Check sheet for the modelled part. Datum: model origin and axes. Units: mm. A direction names the side the tool comes from. Give positions to 0.01 mm unless a question says otherwise; leave off trailing zeros. Loops run counter-clockwise (first coordinate to the right, second up) from the corner with the lowest first, then second, coordinate; pieces in that order, holes last. Notation, with made-up numbers: (-40, -38) - (-7, -38) arc R17 cw to (-7, -11) - close; hole circle Ø3 at (80, -12). An arc over 180 degrees is marked (long way). Use one line per item in the form item = value.
from build123d import *

# Parameters (mm, degrees)
F0_W         = 1.8
F0_H         = 50
F0_W_2       = 18.2
F0_W_3       = 1.6
F1_DEPTH     = 1
F2_DEPTH     = 20
F3_DEPTH     = 20
F4_T4_DEPTH  = 76.7042031505
F4_T9_DEPTH  = 76.6048284538
F4_T14_DEPTH = 76.8048284538
F4_T19_DEPTH = 76.7042031505
F4_T24_DEPTH = 76.6048284538
F4_T29_DEPTH = 76.8048284538
F5_R         = 5
F6_R         = 2
F7_R         = 5
F8_SIZE      = 0.5


# Not quite as in the source:
# - a fillet or chamfer that OpenCascade refuses, or shapes differently, is made with other operations: its cross-section is extruded or revolved along the edge and cut away or added


with BuildPart() as f1:
    # F0 (on Top) → F1 (new body)
    with BuildSketch(Plane.XY):
        with Locations((0.9, 25)):
            Rectangle(F0_W, F0_H)
        with Locations((10.9, 25)):
            Rectangle(F0_W_2, F0_H)
        with Locations((20.8, 25)):
            Rectangle(F0_W_3, F0_H)
        with BuildLine():
            Line((21.6, 50), (21.6, 0))
            Line((21.6, 0), (32.3006253033, 0))
            ThreePointArc((32.3006253033, 0), (36.6893218813, 25), (32.3006253033, 50))
            Line((32.3006253033, 50), (21.6, 50))
        make_face()
        with BuildLine():
            ThreePointArc((32.3006253033, 50), (36.6893218813, 25), (32.3006253033, 0))
            Line((32.3006253033, 0), (34, 0))
            ThreePointArc((34, 0), (38.2893218813, 25), (34, 50))
            Line((34, 50), (32.3006253033, 50))
        make_face()
    extrude(amount=F1_DEPTH)

    # F0 (on Top) → F2 (join)
    with BuildSketch(Plane.XY):
        with Locations((0.9, 25)):
            Rectangle(F0_W, F0_H)
        with Locations((20.8, 25)):
            Rectangle(F0_W_3, F0_H)
    extrude(amount=F2_DEPTH)

    # F0 (on Top) → F3 (join)
    with BuildSketch(Plane.XY):
        with BuildLine():
            ThreePointArc((32.3006253033, 50), (36.6893218813, 25), (32.3006253033, 0))
            Line((32.3006253033, 0), (34, 0))
            ThreePointArc((34, 0), (38.2893218813, 25), (34, 50))
            Line((34, 50), (32.3006253033, 50))
        make_face()
    extrude(amount=F3_DEPTH)

    # F4: fillet of radius 15 on 6 edges, made by hand


with BuildPart() as f4_tool2:
    # F4_s3 → F4_t4 (new body)
    with BuildSketch(Plane.YZ.offset(-5.2017889236)):
        with BuildLine():
            ThreePointArc((15.0009656854, 20.0004), (4.3933982822, 15.6066017178), (-0.0004, 4.9990343146))
            Line((-0.0004, 4.9990343146), (-1.5005365685, 4.9990343146))
            ThreePointArc((-1.5005365685, 4.9990343146), (-1.5001365685, 12.4995171573), (-1.5001365685, 20))
            Line((-1.5001365685, 20), (0, 21.5001365685))
            ThreePointArc((0, 21.5001365685), (7.5004828427, 21.5001365685), (15.0009656854, 21.5005365685))
            Line((15.0009656854, 21.5005365685), (15.0009656854, 20.0004))
        make_face()
    extrude(amount=F4_T4_DEPTH)

    split(bisect_by=Plane.YZ.offset(21.6), keep=Keep.TOP)


with BuildPart() as f1_1:
    add(f1.part)

    # F4_t1: cut F4_tool2
    add(f4_tool2.part, mode=Mode.SUBTRACT)


with BuildPart() as f4_tool7:
    # F4_s8 → F4_t9 (new body)
    with BuildSketch(Plane.YZ.offset(-17.5024142269)):
        with BuildLine():
            ThreePointArc((15.0009656854, 20.0004), (4.3933982822, 15.6066017178), (-0.0004, 4.9990343146))
            Line((-0.0004, 4.9990343146), (-1.5005365685, 4.9990343146))
            ThreePointArc((-1.5005365685, 4.9990343146), (-1.5001365685, 12.4995171573), (-1.5001365685, 20))
            Line((-1.5001365685, 20), (0, 21.5001365685))
            ThreePointArc((0, 21.5001365685), (7.5004828427, 21.5001365685), (15.0009656854, 21.5005365685))
            Line((15.0009656854, 21.5005365685), (15.0009656854, 20.0004))
        make_face()
    extrude(amount=F4_T9_DEPTH)

    split(bisect_by=Plane.YZ.offset(21.6), keep=Keep.TOP)


with BuildPart() as f1_2:
    add(f1_1.part)

    # F4_t6: cut F4_tool7
    add(f4_tool7.part, mode=Mode.SUBTRACT)


with BuildPart() as f4_tool12:
    # F4_s13 → F4_t14 (new body)
    with BuildSketch(Plane.YZ.offset(-37.5024142269)):
        with BuildLine():
            ThreePointArc((-0.0004, 4.9990343146), (4.3933982822, 15.6066017178), (15.0009656854, 20.0004))
            Line((15.0009656854, 20.0004), (15.0009656854, 21.5005365685))
            ThreePointArc((15.0009656854, 21.5005365685), (7.5004828427, 21.5001365685), (0, 21.5001365685))
            Line((0, 21.5001365685), (-1.5001365685, 20))
            ThreePointArc((-1.5001365685, 20), (-1.5001365685, 12.4995171573), (-1.5005365685, 4.9990343146))
            Line((-1.5005365685, 4.9990343146), (-0.0004, 4.9990343146))
        make_face()
    extrude(amount=F4_T14_DEPTH)

    split(bisect_by=Plane.YZ.offset(21.6), keep=Keep.TOP)


with BuildPart() as f1_3:
    add(f1_2.part)

    # F4_t11: cut F4_tool12
    add(f4_tool12.part, mode=Mode.SUBTRACT)


with BuildPart() as f4_tool17:
    # F4_s18 → F4_t19 (new body)
    with BuildSketch(Plane.YZ.offset(71.5024142269)):
        with BuildLine():
            ThreePointArc((34.9990343146, 20.0004), (45.6066017178, 15.6066017178), (50.0004, 4.9990343146))
            Line((50.0004, 4.9990343146), (51.5005365685, 4.9990343146))
            ThreePointArc((51.5005365685, 4.9990343146), (51.5001365685, 12.4995171573), (51.5001365685, 20))
            Line((51.5001365685, 20), (50, 21.5001365685))
            ThreePointArc((50, 21.5001365685), (42.4995171573, 21.5001365685), (34.9990343146, 21.5005365685))
            Line((34.9990343146, 21.5005365685), (34.9990343146, 20.0004))
        make_face()
    extrude(amount=-F4_T19_DEPTH)

    split(bisect_by=Plane.YZ.offset(21.6), keep=Keep.TOP)


with BuildPart() as f1_4:
    add(f1_3.part)

    # F4_t16: cut F4_tool17
    add(f4_tool17.part, mode=Mode.SUBTRACT)


with BuildPart() as f4_tool22:
    # F4_s23 → F4_t24 (new body)
    with BuildSketch(Plane.YZ.offset(59.1024142269)):
        with BuildLine():
            ThreePointArc((34.9990343146, 20.0004), (45.6066017178, 15.6066017178), (50.0004, 4.9990343146))
            Line((50.0004, 4.9990343146), (51.5005365685, 4.9990343146))
            ThreePointArc((51.5005365685, 4.9990343146), (51.5001365685, 12.4995171573), (51.5001365685, 20))
            Line((51.5001365685, 20), (50, 21.5001365685))
            ThreePointArc((50, 21.5001365685), (42.4995171573, 21.5001365685), (34.9990343146, 21.5005365685))
            Line((34.9990343146, 21.5005365685), (34.9990343146, 20.0004))
        make_face()
    extrude(amount=-F4_T24_DEPTH)

    split(bisect_by=Plane.YZ.offset(21.6), keep=Keep.TOP)


with BuildPart() as f1_5:
    add(f1_4.part)

    # F4_t21: cut F4_tool22
    add(f4_tool22.part, mode=Mode.SUBTRACT)


with BuildPart() as f4_tool27:
    # F4_s28 → F4_t29 (new body)
    with BuildSketch(Plane.YZ.offset(39.3024142269)):
        with BuildLine():
            ThreePointArc((34.9990343146, 20.0004), (45.6066017178, 15.6066017178), (50.0004, 4.9990343146))
            Line((50.0004, 4.9990343146), (51.5005365685, 4.9990343146))
            ThreePointArc((51.5005365685, 4.9990343146), (51.5001365685, 12.4995171573), (51.5001365685, 20))
            Line((51.5001365685, 20), (50, 21.5001365685))
            ThreePointArc((50, 21.5001365685), (42.4995171573, 21.5001365685), (34.9990343146, 21.5005365685))
            Line((34.9990343146, 21.5005365685), (34.9990343146, 20.0004))
        make_face()
    extrude(amount=-F4_T29_DEPTH)

    split(bisect_by=Plane.YZ.offset(21.6), keep=Keep.TOP)


with BuildPart() as f1_6:
    add(f1_5.part)

    # F4_t26: cut F4_tool27
    add(f4_tool27.part, mode=Mode.SUBTRACT)

    # F5
    f5_edges = [f1_6.edges().sort_by_distance(p)[0] for p in [
        (36.689322, 25, 1),
        (21.6, 25, 1),
    ]]
    fillet(f5_edges, radius=F5_R)

    # F6
    f6_edges = [f1_6.edges().sort_by_distance(p)[0] for p in [
        (1.8, 25, 1),
        (20, 25, 1),
    ]]
    fillet(f6_edges, radius=F6_R)

    # F7
    f7_edges = [f1_6.edges().sort_by_distance(p)[0] for p in [
        (0.9, 0, 20),
        (20.8, 0, 20),
        (20.8, 50, 20),
        (0.9, 50, 20),
    ]]
    fillet(f7_edges, radius=F7_R)

    # F8
    f8_edges = [f1_6.edges().sort_by_distance(p)[0] for p in [
        (0, 25, 0),
        (17, 0, 0),
        (38.289322, 25, 0),
        (17, 50, 0),
    ]]
    chamfer(f8_edges, length=F8_SIZE)


solid = f1_6.part
Item 1: Section check A-A on z = 14.25. Record the boundary of the cut face in (x, y).
Answer block:
outline = (0, 0) - (1.8, 0) - (1.8, 50) - (0, 50) - close; (20, 0) - (21.6, 0) - (21.6, 50) - (20, 50) - close; (33.37, 3.19) - (35.05, 3.19) arc R75 ccw to (35.05, 46.81) - (33.37, 46.81) arc R73.4 cw to start
Item 2: Thickness scan on L1, parallel to X at y = 24, z = 14; L2, parallel to X at y = 43, z = 15.5; L3, parallel to Z at x = 12, y = 30. Record the ranges inside material, lowest first.
Answer block:
L1 = 0 to 1.8, 20 to 21.6, 36.68 to 38.28
L2 = 0 to 1.8, 20 to 21.6, 34.45 to 36.1
L3 = 0 to 1
Item 3: Section check C-C on z = 11. Record the boundary of the cut face in (x, y).
Answer block:
outline = (0, 0) - (1.8, 0) - (1.8, 50) - (0, 50) - close; (20, 0) - (21.6, 0) - (21.6, 50) - (20, 50) - close; (32.74, 1.25) - (34.43, 1.25) arc R75 ccw to (34.43, 48.75) - (32.74, 48.75) arc R73.4 cw to start
Item 4: Section check B-B on x = 22.5. Record the boundary of the cut face in (y, z).
Answer block:
outline = (0, 0.5) - (0.5, 0) - (49.5, 0) - (50, 0.5) - (50, 3.14) - (0, 3.14) - close
Item 5: Mould release check, pull along X, two halves, no side actions. Record for faces 5 (the face through (21, 48, 19)), 6 (the face through (1.8, 25, 11)), 7 (the face through (37.924, 24.645, 0.135)): released by +X, released by -X, zero draft, split by the parting line, or undercut.
Answer block:
face_5 = zero draft
face_6 = undercut
face_7 = released by +X
Item 6: Gauge pin test, flat ends, axial feed: P1, Ø6, axis at x = 12.5, z = 6, coming from the +Y side; P2, Ø2, axis at x = 14.5, y = 10, coming from the +Z side; P3, Ø8, axis at y = 39.5, z = 3.5, coming from the +X side. Record the tip position at first contact, or that the pin passes through.
Answer block:
P1 = through
P2 = 1
P3 = 37.55
Item 7: Access from +Z, -Z, +X, -X, +Y, -Y to the whole of each face (thin tool, end or side, straight path). Record for faces 1 (the face through (29, 25, 1)), 2 (the face through (34.498, 4.432, 15.645)), 3 (the face through (11, 25, 1)), 4 (the face through (34.923, 45.568, 15.645)).
Answer block:
face_1 = +Z
face_2 = +Z, +X, -Y
face_3 = +Z, +Y, -Y
face_4 = +Z, +X, +Y
